Geometry check sheet. Reference: drawing and pictorial views, mm from the part's lowest x, y, z. Coordinates: 2 decimals unless noted, no trailing zeros. Answer as CSV lines item,"result". Start each with the question number.
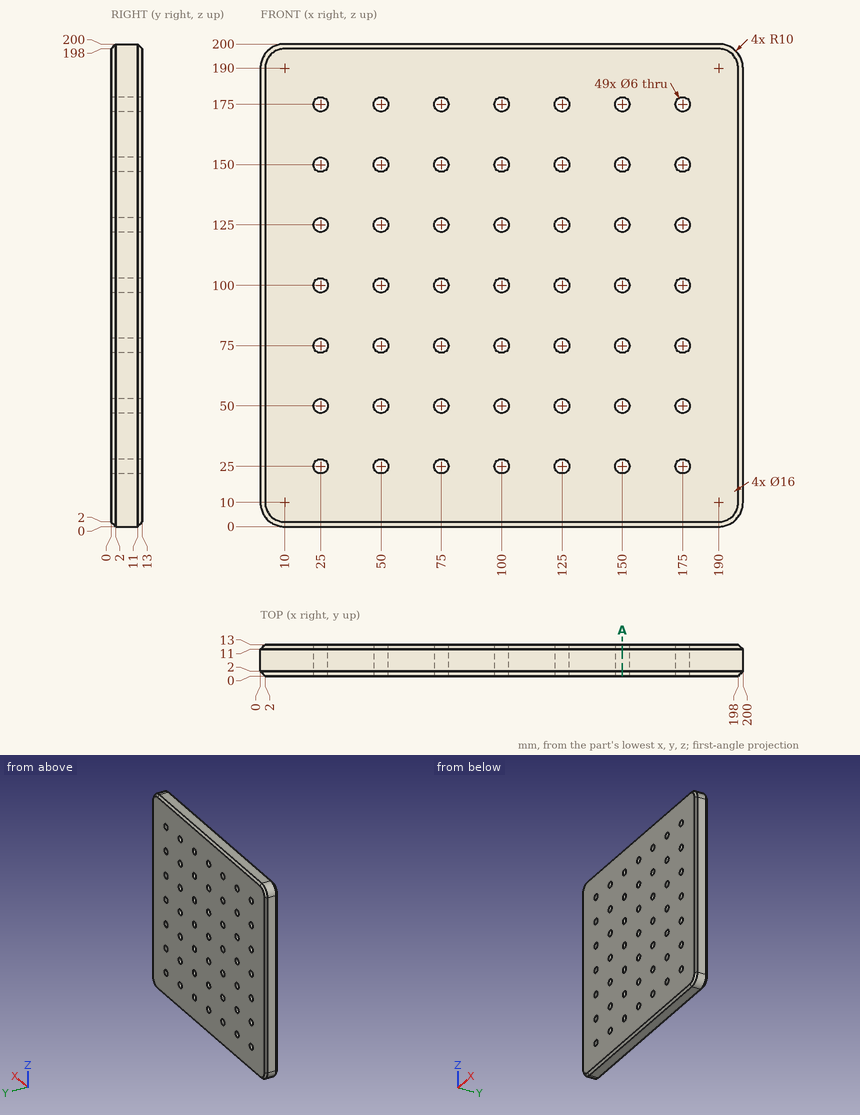
1. Cross-section at A-A (x = 150). Count the separate pieces of the cut face and the enclosed holes in it, and give its area (3 significant figures).
2. Depth check by flat-ended pin: P1, Ø5.5, axis at x = 75, z = 100, coming from the +Y side. Enter the tip coordinate at first touch or a pass-through.
3. Scan lines: line 1 along Z through (x, y) = (60, 1.75); line 2 along X through (y, z) = (12.25, 66.5); line 3 along X through (y, z) = (11.5, 183). Record each from-to range of solid material in increasing order. Write a range as from..to.
Completed:
1,separate pieces,"8"
1,enclosed holes,"0"
1,area,"2,050 mm2"
2,P1,"passes through"
3,line 1,"z = 0.25..199.75"
3,line 2,"x = 1.25..198.75"
3,line 3,"x = 0.5..199.5"
